```python
from build123d import *

# Parameters (mm, degrees)
SKETCH1_R           = 7.5
BOSS_EXTRUDE1_DEPTH = 2


with BuildPart() as part:
    # Sketch1 → Boss-Extrude1 (new body)
    with BuildSketch(Plane.XY):
        Polygon((-73, -24), (21, -24), (49.284271247, 4.284271247), (83.091675168, 13.342937826), (97.844360738, 68.400709925), (22.500150609, 111.900709925), (-20.633363043, 68.767196272), (-33.056677208, 22.40275661), (-115.160372443, 44.402375444), (-101.442963052, -6.791693349), align=None)
        Circle(SKETCH1_R, mode=Mode.SUBTRACT)
        with Locations((-73, 0)):
            Circle(SKETCH1_R, mode=Mode.SUBTRACT)
        with BuildLine():
            Line((64.520092973, 55.334506438), (58.308435891, 32.152286607))
            ThreePointArc((58.308435891, 32.152286607), (49.122849355, 26.848985748), (43.819548496, 36.034572283))
            Line((43.819548496, 36.034572283), (50.031205579, 59.216792114))
            ThreePointArc((50.031205579, 59.216792114), (59.216792114, 64.520092973), (64.520092973, 55.334506438))
        make_face(mode=Mode.SUBTRACT)
    extrude(amount=BOSS_EXTRUDE1_DEPTH)


solid = part.part
```
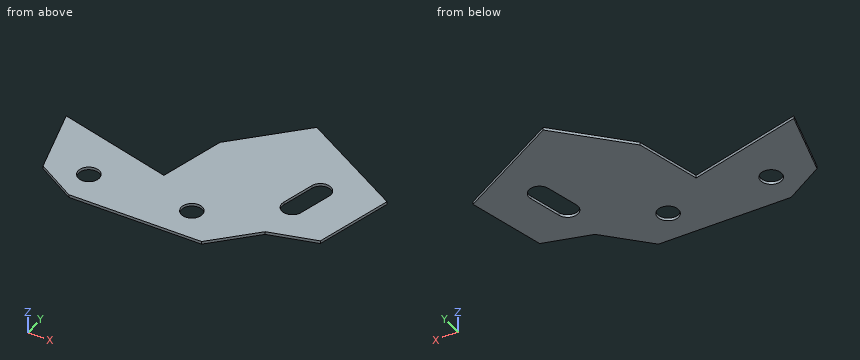
Source: CAD feature listing. Evaluate the final solid. Frame: model axes, mm. Give positions to 0.01 mm unless a question says otherwise; leave off trailing zeros. Order: outer loops, then holes, each group sorted by start corner. A loop starts at its lowest first (then second) coordinate and runs counter-clockwise, first axis right, second up. Notation, with made-up numbers: (-5.5, 21.25) -> (37.5, 21.25) arc R31 cw to (37.5, 55.25) -> close; hole circle Ø7 at (20.25, -3.75). An arc over 180 degrees is marked (long way). Use a Markdown table: item, result.
Q1. Section A-A (z = 1.1). Return the cut outline in (x, y), and give its area (3 significant figures).
A:
| item | result |
|---|---|
| outline | (-115.16, 44.4) -> (-101.44, -6.79) -> (-73, -24) -> (21, -24) -> (49.28, 4.28) -> (83.09, 13.34) -> (97.84, 68.4) -> (22.5, 111.9) -> (-20.63, 68.77) -> (-33.06, 22.4) -> close; hole circle Ø15 at (-73, 0); hole circle Ø15 at (0, 0); hole (43.82, 36.03) arc R7.5 ccw to (58.31, 32.15) -> (64.52, 55.33) arc R7.5 ccw to (50.03, 59.22) -> close |
| area | 14,900 mm^2 |
Q2. Material intervals for line 1 (X direction, y = -1.5, z = 1.4); line 2 (Y direction, x = -73, z = 1.3); line 3 (Y direction, x = 0, z = 1.4), sorted ascending. Write a range as [from, to].
A:
| item | result |
|---|---|
| line 1 | [-102.86, -80.35], [-65.65, -7.35], [7.35, 43.5] |
| line 2 | [-24, -7.5], [7.5, 33.11] |
| line 3 | [-24, -7.5], [7.5, 89.4] |
Q3. Section D-D (y = 100). Return the cut outline in (x, z).
A:
| item | result |
|---|---|
| outline | (10.6, 0) -> (43.11, 0) -> (43.11, 2) -> (10.6, 2) -> close |
Q4. Section B-B (y = 0). Return the cut outline in (x, z).
A:
| item | result |
|---|---|
| outline | (-103.26, 0) -> (-80.5, 0) -> (-80.5, 2) -> (-103.26, 2) -> close; (-65.5, 0) -> (-7.5, 0) -> (-7.5, 2) -> (-65.5, 2) -> close; (7.5, 0) -> (45, 0) -> (45, 2) -> (7.5, 2) -> close |
Q5. Section C-C (x = 0). Return the cut outline in (y, z), and give its area (3 significant figures).
A:
| item | result |
|---|---|
| outline | (-24, 0) -> (-7.5, 0) -> (-7.5, 2) -> (-24, 2) -> close; (7.5, 0) -> (89.4, 0) -> (89.4, 2) -> (7.5, 2) -> close |
| area | 197 mm^2 |
Q6. First-contact query: P1, Ø1, axis at y = 78, z = 0.5, coming from the +X side; P2, Ø5, axis at x = 38, y = 48, coming from the -Z side; P3, Ø12, axis at x = 0, y = 0, coming from the +Z side. Flat tips, straight axial feed; report the tip coordinate or a pass-through.
A:
| item | result |
|---|---|
| P1 | x = 82.08 |
| P2 | z = 0 |
| P3 | through |
